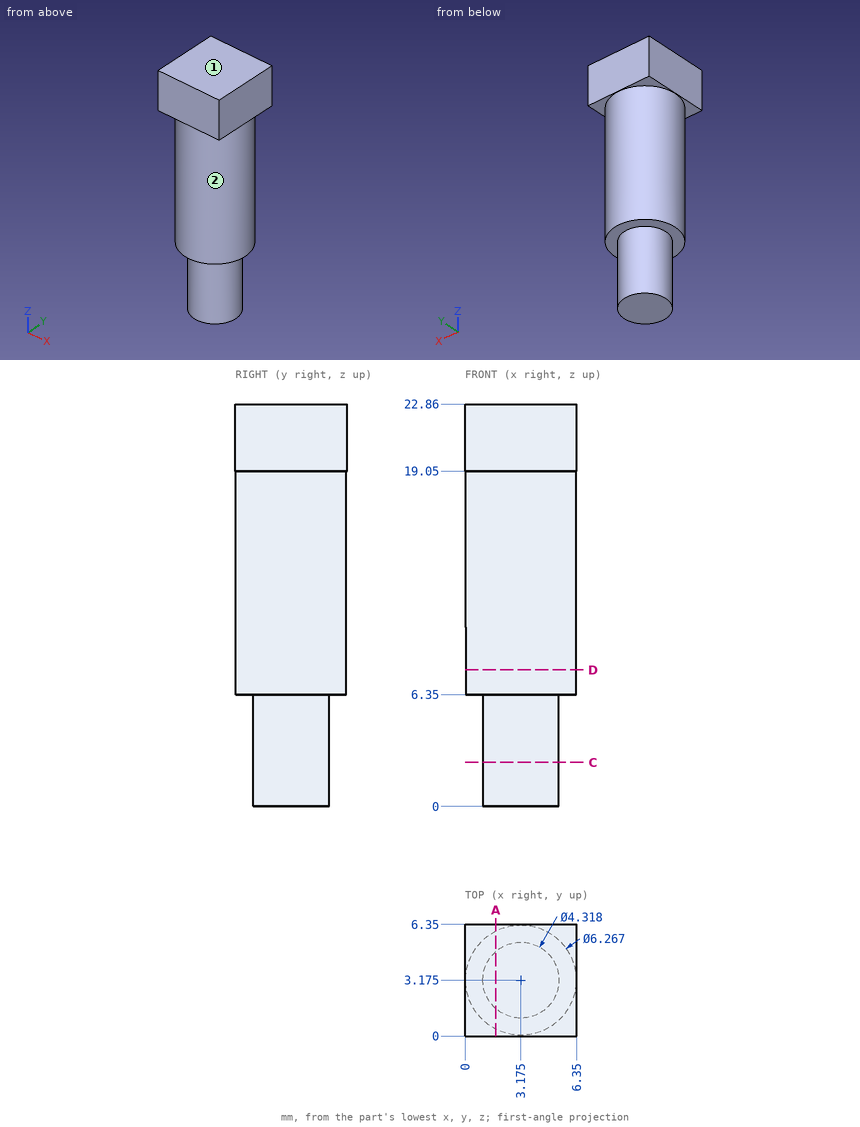
Part print with two shaded views. Sizes in mm from the minimum x, y, z corner. A direction names the side the tool comes from. Coordinates: 2 decimals unless noted, no trailing zeros. Order: outer loops, then holes, each group sorted by start corner. A loop starts at its lowest first (then second) coordinate and runs counter-clockwise, first axis right, second up.
(1) Which spindle directions (+Z, -Z, +X, -X, +Y, -Y) get a long thin tool onto all of the face, cutting with end or side? Do the marked faces 1 and 2. Say none if no direction does.
Solution:
face 1: +Z, +X, -X, +Y, -Y
face 2: -Z
(2) Pin check, flat tips, straight feed: pin 1 Ø2 at (x, y) = (5.5, 2) entering from -Z; pin 2 Ø1.5 at (y, z) = (3.5, 8.5) entering from +X. Stop position of each tip, or through.
Solution:
pin 1: stops at z = 0
pin 2: stops at x = 6.31
(3) Drill centre lines: L1, parallel to Z at x = 3.75, y = 1; L2, parallel to X at y = 1.5, z = 7.75 (1 decimal); L3, parallel to Y at x = 3.75, z = 11.75 (1 decimal). Where is each one in solid material? Low to high.
Solution:
L1: z = 6.35 to 22.86
L2: x = 0.5 to 5.8
L3: y = 0.1 to 6.3
(4) Saw through at C-C, the plane z = 2.5. Write the cut outline in (x, y) (1 decimal).
Solution:
outline: circle Ø4.3 at (3.2, 3.2)
(5) Saw through at D-D, the plane z = 7.75. Write the cut outline in (x, y) (1 decimal).
Solution:
outline: circle Ø6.3 at (3.2, 3.2)
(6) Saw through at A-A, the plane x = 1.75. Write the cut outline in (y, z).
Solution:
outline: (0, 19.05) - (0.38, 19.05) - (0.38, 6.35) - (1.55, 6.35) - (1.55, 0) - (4.8, 0) - (4.8, 6.35) - (5.97, 6.35) - (5.97, 19.05) - (6.35, 19.05) - (6.35, 22.86) - (0, 22.86) - close
